Check sheet for the drawn part. Datum: minimum x, y, z corner. Units: mm. A direction names the side the tool comes from. Give positions to 0.01 mm unless a question says otherwise; leave off trailing zeros. Write each loop counter-clockwise with the first axis right and the second up, starting at its lowest first coordinate (ties: lowest second). Pieces come first, ordered by that corner, then holes.
(1) Mould release check, pull along X, two halves, no side actions. Record for the marked faces 3, 4, 5 and 6: +X half, -X half, draft (parallel to the pull), parting line (faces both ways), or undercut.
(2) Tool access check on the marked faces 1 and 2. Record the directions out of +Z, -Z, +X, -X, +Y, -Y that give a thin tool (end or side, any length) a straight path to the whole face; none if there is none.
(3) Depth check by flat-ended pin: P1, Ø2, axis at y = 7.5, z = 6.5, coming from the -X side (1 decimal); P2, Ø1.5, axis at y = 15.5, z = 9, coming from the -X side; P3, Ø2.5, axis at y = 4.5, z = 1, coming from the -X side (1 decimal). Enter the tip coordinate at first touch or a pass-through.
(4) Cross-section at D-D (z = 4.75). Record the boundary of the cut face in (x, y).
(5) Cross-section at C-C (z = 9). Record the boundary of the cut face in (x, y), and give its area (3 significant figures).
(6) Thickness scan on line 1 along X through (y, z) = (9.5, 1.2); line 2 along Y through (x, z) = (9.5, 4.5); line 3 along Y through (x, z) = (9.5, 8.25). Record the ranges inside material, lowest first.
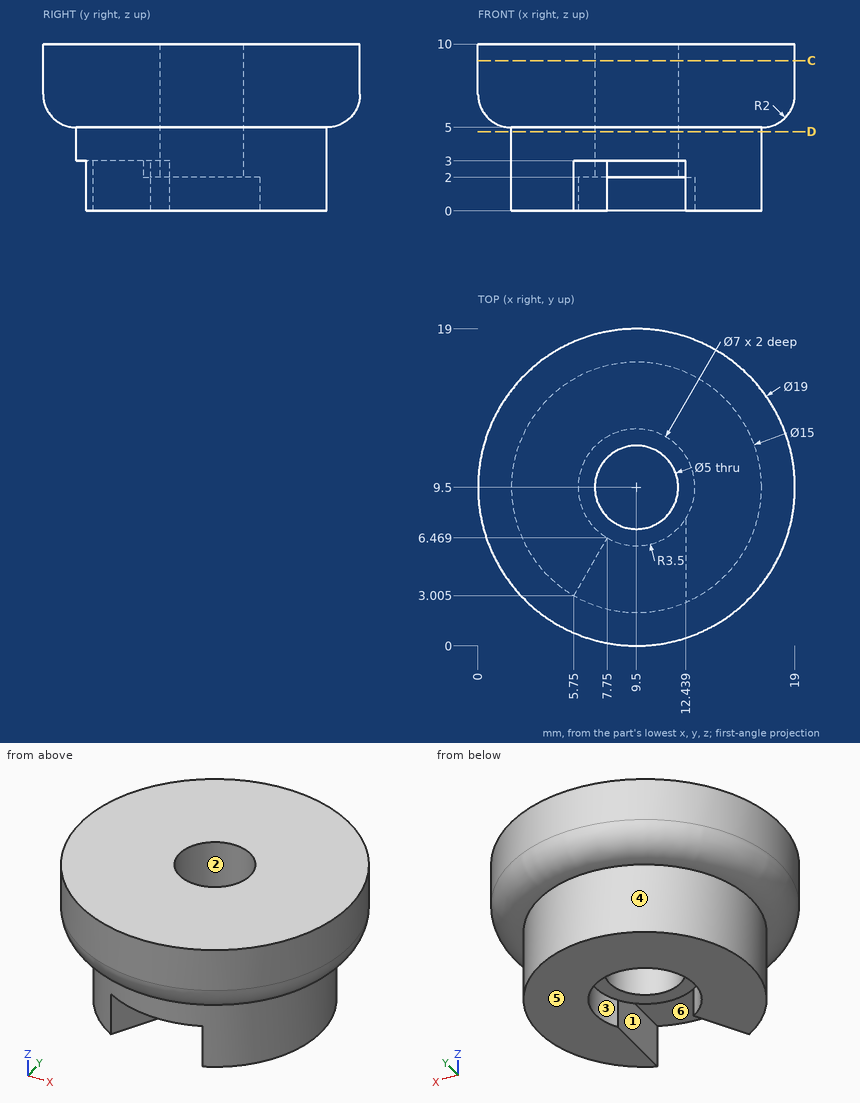
Reply:
1. face 3: undercut
1. face 4: parting line
1. face 5: draft
1. face 6: undercut
2. face 1: -Z, -Y
2. face 2: +Z, -Z
3. P1: stops at x = 0.1
3. P2: stops at x = 1.58
3. P3: stops at x = 3
4. outline: circle Ø15 at (9.5, 9.5); hole circle Ø5 at (9.5, 9.5)
5. outline: circle Ø19 at (9.5, 9.5); hole circle Ø5 at (9.5, 9.5)
5. area: 264 mm2
6. line 1: x = 2 to 6, 13 to 17
6. line 2: y = 2 to 7, 12 to 17
6. line 3: y = 0 to 7, 12 to 19
